Model file for the job. Use its own axes, mm. A direction names the side the tool comes from. Give positions to 0.01 mm unless a question says otherwise; leave off trailing zeros. Order: outer loops, then holes, each group sorted by start corner. A loop starts at its lowest first (then second) coordinate and runs counter-clockwise, first axis right, second up. Notation, with made-up numbers: M 27,-38.75 L 57,-38.75 A11 cw 57,-22.75 Z; hole C 42,54 d7. An arc over 180 degrees is marked long. Return JSON: item names as keys, results as strings. Group by question number.
1. Two-plate mould, pull along X, no slides. Class faces 1 (the face through (29, 0, 0)), 2 (the face through (31, -19, 9.525)): released by +X, released by -X, zero draft, split by the parting line, or undercut.
2. Slice it at D-D on x = -21. List the corners of the cut face in (y, z) (3 decimals), then the cut area to 3 significant figures.
3. Wall check: probe 1 along X at (y, z) = (-16, 1); probe 2 along X at (y, z) = (-7, 3); probe 3 along Z at (x, y) = (101.5, -7) (3 decimals). Give the ranges that are in metal, low to high. Write a range as [from, to].
4. Slice it at A-A on y = -14.5. List the corners of the cut face in (x, z) (3 decimals).
5. Pin check, flat tips, straight feed: pin 1 (10 mm diameter, centred on x = 0, y = -26.5, fed in from +Z) (3 decimals); pin 2 (3 mm diameter, centred on x = 86, y = -6, fed in from -Z) (3 decimals); pin 3 (3 mm diameter, centred on y = -31.5, z = -14.5, fed in from -X). Stop position of each tip, or through.
6. Slice it at C-C on z = -7.5. List the corners of the cut face in (x, y), then the cut area to 3 significant figures.
7. 3-axis set-ups, long thin cutter, end or side, ignore diameter. For faces 3 (the face through (-80.836, -18.783, 0.698)), 4 (the face through (29, -19, -9.525)): which of +Z, -Z, +X, -X, +Y, -Y reach the whole face in a straight line?
8. Slice it at B-B on x = 115.5. List the corners of the cut face in (y, z), then the cut area to 3 significant figures.
from build123d import *

# Parameters (mm, degrees)
F0_R     = 12.7
F0_W     = 1.2455678842
F0_H     = 19.05
F1_DEPTH = 38.1


with BuildPart() as f1:
    # F0 (on Front) → F1 (new body)
    with BuildSketch(Plane.XZ):
        with BuildLine():
            ThreePointArc((-45.300738686, -9.525), (-43.3976356373, -4.9305028092), (-42.7485226281, 0))
            ThreePointArc((-42.7485226281, 0), (-43.3976356373, 4.9305028092), (-45.300738686, 9.525))
            Line((-45.300738686, 9.525), (-45.300738686, -9.525))
        make_face()
        with BuildLine():
            ThreePointArc((-45.300738686, 9.525), (-43.3976356373, 4.9305028092), (-42.7485226281, 0))
            ThreePointArc((-42.7485226281, 0), (-43.3976356373, -4.9305028092), (-45.300738686, -9.525))
            Line((-45.300738686, -9.525), (105.8536934298, -9.525))
            ThreePointArc((105.8536934298, -9.525), (103.3014773719, 0), (105.8536934298, 9.525))
            Line((105.8536934298, 9.525), (-45.300738686, 9.525))
        make_face()
        with BuildLine():
            Line((-46.5463065702, 9.525), (-45.300738686, 9.525))
            ThreePointArc((-45.300738686, 9.525), (-80.8485226281, 0), (-45.300738686, -9.525))
            Line((-45.300738686, -9.525), (-46.5463065702, -9.525))
            Line((-46.5463065702, -9.525), (-46.5463065702, 9.525))
        make_face()
        with Locations((-61.7985226281, 0)):
            Circle(F0_R, mode=Mode.SUBTRACT)
        with Locations((-45.9235226281, 0)):
            Rectangle(F0_W, F0_H)
        with BuildLine():
            ThreePointArc((141.4014773719, 0), (127.2819801811, 18.4008869908), (105.8536934298, 9.525))
            Line((105.8536934298, 9.525), (107.099261314, 9.525))
            Line((107.099261314, 9.525), (107.099261314, -9.525))
            Line((107.099261314, -9.525), (105.8536934298, -9.525))
            ThreePointArc((105.8536934298, -9.525), (127.2819801811, -18.4008869908), (141.4014773719, 0))
        make_face()
        with Locations((122.3514773719, 0)):
            Circle(F0_R, mode=Mode.SUBTRACT)
        with BuildLine():
            Line((105.8536934298, -9.525), (105.8536934298, 9.525))
            ThreePointArc((105.8536934298, 9.525), (103.3014773719, 0), (105.8536934298, -9.525))
        make_face()
        with Locations((106.4764773719, 0)):
            Rectangle(F0_W, F0_H)
    extrude(amount=F1_DEPTH)


solid = f1.part
Result:
{
 "1": {"face 1": "zero draft", "face 2": "undercut"},
 "2": {"outline": "M -38.1,-9.525 L 0,-9.525 L 0,9.525 L -38.1,9.525 Z", "area": "726 mm2"},
 "3": {"probe 1": "x = [-80.82, -74.46], [-49.14, 109.69], [135.01, 141.38]", "probe 2": "x = [-80.61, -74.14], [-49.46, 110.01], [134.69, 141.16]", "probe 3": "z = [-9.525, 9.525]"},
 "4": {"outline": "M -45.301,-9.525 L 105.854,-9.525 A19.05 ccw long 105.854,9.525 L -45.301,9.525 A19.05 ccw long Z; hole C -61.799,0 d25.4; hole C 122.351,0 d25.4"},
 "5": {"pin 1": "stops at z = 9.525", "pin 2": "stops at z = -9.525", "pin 3": "stops at x = -75.72"},
 "6": {"outline": "M -79.31,-38.1 L -72.05,-38.1 L -72.05,0 L -79.31,0 Z; M -51.55,-38.1 L 112.1,-38.1 L 112.1,0 L -51.55,0 Z; M 132.6,-38.1 L 139.86,-38.1 L 139.86,0 L 132.6,0 Z", "area": "6,790 mm2"},
 "7": {"face 3": "+Y, -Y", "face 4": "-Z, +Y, -Y"},
 "8": {"outline": "M -38.1,-17.78 L 0,-17.78 L 0,-10.69 L -38.1,-10.69 Z; M -38.1,10.69 L 0,10.69 L 0,17.78 L -38.1,17.78 Z", "area": "540 mm2"}
}
